Verification items for this drawing (mm, ordinates from the low corner). Round coordinates to 2 decimals unless told otherwise and drop trailing zeros. Write each loop counter-clockwise with the first axis right and the second up, starting at its lowest first coordinate (ties: lowest second). Pieces come first, ordered by that corner, then holes.
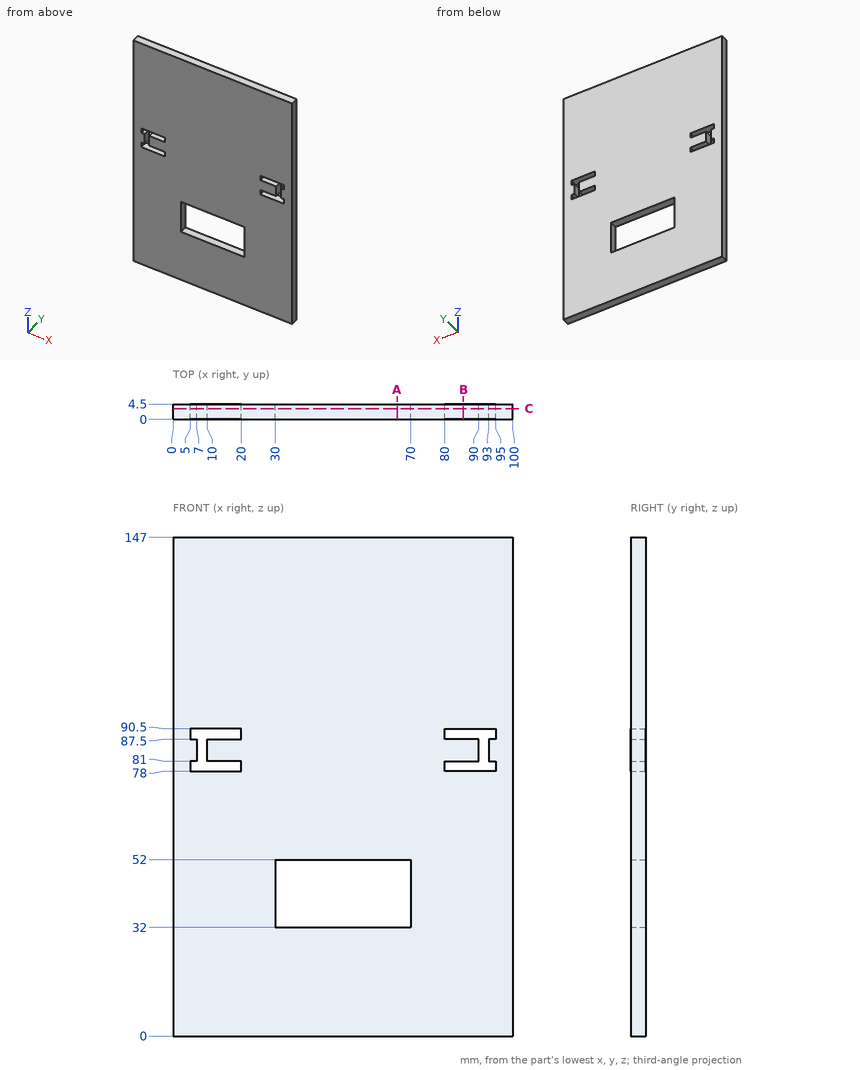
1. Scan lines: line 1 along X through (y, z) = (0.2, 80.5); line 2 along Z through (x, y) = (6, 0.5); line 3 along Z through (x, y) = (91.5, 0.4). Record each from-to range of solid material in increasing order.
2. Section check A-A (x = 66). Record the cut outline in (y, z), plus the area to 4 significant figures.
3. Depth check by flat-ended pin: pin 1 Ø8 at (x, z) = (23.5, 67) entering from -Y. Enter the tip coordinate at first touch or a pass-through.
4. Section check C-C (y = 3.15). State how many separate pieces and enclosed holes the cut face has, plus the area to 3 significant figures.
5. Section check B-B (x = 85.5). Record the cut outline in (y, z), plus the area to 4 significant figures.
Results below:
1. line 1: x = 0 to 5, 20 to 80, 95 to 100
1. line 2: z = 0 to 78, 81 to 87.5, 90.5 to 147
1. line 3: z = 0 to 78, 90.5 to 147
2. outline: (0, 0) - (4.5, 0) - (4.5, 32) - (0, 32) - close; (0, 52) - (4.5, 52) - (4.5, 147) - (0, 147) - close
2. area: 571.5 mm2
3. pin 1: stops at y = 0
4. separate pieces: 1
4. enclosed holes: 3
4. area: 13,700 mm2
5. outline: (0, 0) - (4.5, 0) - (4.5, 78) - (0, 78) - close; (0, 81) - (4.5, 81) - (4.5, 87.5) - (0, 87.5) - close; (0, 90.5) - (4.5, 90.5) - (4.5, 147) - (0, 147) - close
5. area: 634.5 mm2
